Autodesk Inventor part; units mm, degrees
ref_plane "YZ Plane" through (0, 0, 0) normal (1, 0, 0) x (0, 1, 0)
ref_plane "XZ Plane" through (0, 0, 0) normal (0, 1, 0) x (-1, 0, 0)
ref_plane "XY Plane" through (0, 0, 0) normal (0, 0, 1) x (1, 0, 0)
sketch "Эскиз1" plane through (0, 0, 0) normal (0, 1, 0) x (-1, 0, 0)
  line L0 (2.3, 2.625) -> (-2.3, 2.625) construction
  line L1 (-2.3, 2.625) -> (-2.3, -2.625)
  line L2 (-2.3, -2.625) -> (2.3, -2.625)
  line L3 (2.3, -2.625) -> (2.3, 2.625)
  line L4 (3.22, 0) -> (-3.22, 0)
  line L5 (0, -3.7758) -> (0, 4.2798)
  arc A0 (2.3, 2.625) -> (-2.3, 2.625) centre (0, -2.371) ccw
  point P0 (0, 0)
  dimension "d0" = 4.6
  dimension "d10" = 5.25
  dimension "d17" = 5.5
extrude "Выдавливание1" add sketch "Эскиз1" along normal blind 5
chamfer "Фаска2" distance 5 angle 45 1 edges at (0, 0, -2.625)
sketch "Эскиз3" plane through (0, 5, 0) normal (0, 1, 0) x (1, 0, 0)
  line L0 (2.3, -2.625) -> (2.3, 2.625)
  line L1 (2.3, 2.625) -> (1.3, 2.625)
  line L2 (1.3, 2.625) -> (1.3, -3.129)
  line L3 (1.3, -3.129) -> (2.3, -3.129)
  line L4 (2.3, -3.129) -> (2.3, 2.625)
  arc A0 (-2.3, -2.625) -> (2.3, -2.625) centre (0, 2.371) ccw
  point P0 (0, 0)
  dimension "d14" = 1
extrude "Выдавливание3" cut sketch "Эскиз3" against normal blind 3
mirror "Зеркальное отражение1" about plane through (0, 0, 0) normal (1, 0, 0) of "Выдавливание3"
sketch "Эскиз4" plane through (0, 5, 0) normal (0, 1, 0) x (1, 0, 0)
  line L0 (-1.3, 2.625) -> (-1.3, -2.9732)
  arc A0 (-1.3, -2.9732) -> (1.3, -2.9732) centre (0, 2.371) ccw
  line L1 (1.3, -2.9732) -> (1.3, 2.625)
  line L2 (1.3, 2.625) -> (-1.3, 2.625)
  point P0 (0, 0)
extrude "Выдавливание4" add sketch "Эскиз4" along normal blind 1
sketch "Эскиз5" plane through (0, 6, 0) normal (0, 1, 0) x (1, 0, 0)
  line L0 (6.5, 2.625) -> (-6.5, 2.625)
  line L1 (1.3, 2.625) -> (-1.3, 2.625)
  line L2 (0, 4.729) -> (0, -4.4387)
  arc A0 (-6.5, 2.625) -> (6.5, 2.625) centre (0, 3.4194) ccw
  arc A1 (-1.3, -2.9732) -> (1.3, -2.9732) centre (0, 2.371) ccw
  point P0 (0, 0)
  point P1 (0, -3.129)
  dimension "d20" = 13
extrude "Выдавливание5" add sketch "Эскиз5" along normal blind 1
properties part number "BUTTON_INSIDE"
Geometry: final body of the model. Coordinates: model frame, mm. A direction names the side the tool comes from. Coordinates: 2 decimals unless noted, no trailing zeros. Loops run counter-clockwise (first coordinate to the right, second up) from the corner with the lowest first, then second, coordinate; pieces in that order, holes last. Notation, with made-up numbers: (3.25, 57.5) - (51.25, 57.5) arc R28 cw to (51.25, 95.5) - close; hole circle Ø3 at (55, 10.25). An arc over 180 degrees is marked (long way). Put each result on its own line as item: value. Start each with the question number.
Q1. Pin query (flat end, axial travel): pin 1 Ø2 at (y, z) = (4, 2.5) entering from -X; pin 2 Ø1.2 at (y, z) = (4.5, 1.5) entering from +X; pin 3 Ø3 at (y, z) = (3, 0.5) entering from -X. Return the tip coordinate at first contact, or that it passes through.
Q2. Set-up query: faces 1 (the flat face through (-2.3, 1, 2)), 2 (the flat face through (1.3, 4, 1)), 3 (the cylindrical face through (0.03, 1.91, 3.13)). Return all of +Z, -Z, +X, -X, +Y, -Y with unobstructed straight access to the full face (end or side cutting, diameter ignored); none if empty.
Q3. Pull-direction query (Y, two-part tool) for faces 4 (the flat face through (0.032, 1.979, 0.395)), 5 (the flat face through (2.3, 1, 2)), 6 (the flat face through (-1.3, 4, 1)), 7 (the flat face through (-2, 2, 2)); classes: released by +Y, released by -Y, zero draft, split by the parting line, or undercut.
Q4. Cut plane A-A, the plane x = -1.5. Return loops of the section in (y, z) (1 decimal).
Q5. Cut plane B-B, the plane z = 0.7. Return loops of the section in (x, y), and give its area (3 significant figures).
Q6. Line query: line 1 (Y direction, x = 3.5, z = 0.2); line 2 (X direction, y = 3.25, z = 1); line 3 (Y direction, x = 1.5, z = 1.7). Output: solid intervals per line, ascending.
Q7. Cut plane C-C, the plane y = 4.5. Return loops of the section in (x, z), and give its area (3 significant figures).
Filled sheet:
1. pin 1: x = -1.3
1. pin 2: x = 1.3
1. pin 3: x = -2.3
2. face 1: +Z, -Z, -X, -Y
2. face 2: +Z, -Z, +X
2. face 3: +Z, -Y
3. face 4: released by -Y
3. face 5: zero draft
3. face 6: undercut
3. face 7: undercut
4. outline: (0, 2.4) - (2, 0.4) - (2, 2.9) - (0, 2.9) - close; (6, -2.6) - (7, -2.6) - (7, 3) - (6, 3) - close
5. outline: (-5.09, 6) - (-1.3, 6) - (-1.3, 2) - (-2.3, 2) - (-2.3, 1.67) - (2.3, 1.67) - (2.3, 2) - (1.3, 2) - (1.3, 6) - (5.09, 6) - (5.09, 7) - (-5.09, 7) - close
5. area: 22.1 mm²
6. line 1: 6 to 7
6. line 2: -1.3 to 1.3
6. line 3: 0.67 to 2, 6 to 7
7. outline: (-1.3, -2.13) - (1.3, -2.13) - (1.3, 2.97) arc R5.5 ccw to (-1.3, 2.97) - close
7. area: 13.5 mm²
